from build123d import *

# Parameters (mm, degrees)
SKETCH1_W                = 76.21
SKETCH1_H                = 100
BOSS_EXTRUDE1_DEPTH      = 5
M4_CLEARANCE_HOLE1_D     = 4.5
M4_CLEARANCE_HOLE1_DEPTH = 5
M4_CLEARANCE_HOLE1_TIP   = 1.351936393


with BuildPart() as part:
    # Sketch1 → Boss-Extrude1 (new body)
    with BuildSketch(Plane.XY):
        with Locations((2.360596056, -12.518477597)):
            Rectangle(SKETCH1_W, SKETCH1_H)
    extrude(amount=BOSS_EXTRUDE1_DEPTH)

    # M4 Clearance Hole1
    with Locations(Plane.XY.offset(5)):
        with Locations((-27.639403944, 7.481522403), (-27.639403944, 27.481522403), (32.360596056, 7.481522403), (32.360596056, 27.481522403), (32.360596056, -52.518477597), (32.360596056, -34.818262245), (-27.639403944, -34.818262245), (-27.639403944, -52.518477597)):
            Hole(M4_CLEARANCE_HOLE1_D / 2, depth=M4_CLEARANCE_HOLE1_DEPTH)
            with Locations((0, 0, -(M4_CLEARANCE_HOLE1_DEPTH + M4_CLEARANCE_HOLE1_TIP / 2))):  # 118° drill point
                Cone(0, M4_CLEARANCE_HOLE1_D / 2, M4_CLEARANCE_HOLE1_TIP, mode=Mode.SUBTRACT)


solid = part.part
The model under review builds one solid part; all positions refer to its coordinate system, in mm. Round coordinates to 2 decimals unless told otherwise and drop trailing zeros. Write each loop counter-clockwise with the first axis right and the second up, starting at its lowest first coordinate (ties: lowest second). Pieces come first, ordered by that corner, then holes. Notation, with made-up numbers: M -38.75,49 L -14.75,49 A23 cw -14.75,82 Z; hole C 64,2 d1. An arc over 180 degrees is marked long. Use a Markdown table: item, result. Add a question column.
Q1. The part is to be moulded in two halves that separate along X. For faces 1 (the face through (-35.744, -13, 2)), 2 (the face through (40.466, -13, 2)), 3 (the face through (-25.854, -53.888, 2.465)), 4 (the face through (2, 37.482, 2)), say which applies: pulls with the +X half, pulls with the -X half, needs draft (parallel to the pull), parting line crosses it, or undercut.
Q2. To check wall thickness, follow line 1 (Y direction, x = -27.5, z = 3.15); line 2 (X direction, y = -51, z = 1.1); line 3 (X direction, y = -36, z = 1.7). State the ranges of each line that lie inside material, in increasing order.
Q3. We need section B-B, the plane z = 3.35. Count the separate pieces of the cut face and the enclosed holes in it, plus the area to 3 significant figures.
Q4. Insertion check: pin 1 (6 mm diameter, centred on x = -27.64, y = 7.48, fed in from +Z); pin 2 (3.5 mm diameter, centred on x = 32.36, y = -52.52, fed in from -Z). Each pin has a flat end and moves straight along its axis. Give the tip position at first contact, or say it passes through.
Q5. We need section A-A, the plane y = -51.5. State the section outline as (x, z) points, plus the area to 3 significant figures.
Findings below:
| question | item | result |
|---|---|---|
| 1 | face 1 | pulls with the -X half |
| 1 | face 2 | pulls with the +X half |
| 1 | face 3 | undercut |
| 1 | face 4 | needs draft |
| 2 | line 1 | y = -62.52 to -54.76, -50.27 to -37.06, -32.57 to 5.24, 9.73 to 25.24, 29.73 to 37.48 |
| 2 | line 2 | x = -35.74 to -29.3, -25.98 to 30.7, 34.02 to 40.47 |
| 2 | line 3 | x = -35.74 to -29.55, -25.72 to 30.45, 34.28 to 40.47 |
| 3 | separate pieces | 1 |
| 3 | enclosed holes | 8 |
| 3 | area | 7,490 mm² |
| 4 | pin 1 | stops at z = 5 |
| 4 | pin 2 | passes through |
| 5 | outline | M -35.74,0 L -29.65,0 L -29.65,5 L -35.74,5 Z; M -25.63,0 L 30.35,0 L 30.35,5 L -25.63,5 Z; M 34.37,0 L 40.47,0 L 40.47,5 L 34.37,5 Z |
| 5 | area | 341 mm² |
